Read the model definition and answer for the solid it produces. Units are mm, in the model's axes. A direction names the side the tool comes from. Coordinates: 2 decimals unless noted, no trailing zeros. Loops run counter-clockwise (first coordinate to the right, second up) from the corner with the lowest first, then second, coordinate; pieces in that order, holes last. Notation, with made-up numbers: (51.5, 22) - (110.5, 22) arc R18 ccw to (110.5, 48) - close; hole circle Ø5 at (-13.75, -19.5). An arc over 180 degrees is marked (long way). Use one line per item in the form item = value.
Autodesk Inventor part; units mm, degrees
ref_plane "YZ Plane" through (0, 0, 0) normal (1, 0, 0) x (0, 1, 0)
ref_plane "XZ Plane" through (0, 0, 0) normal (0, 1, 0) x (-1, 0, 0)
ref_plane "XY Plane" through (0, 0, 0) normal (0, 0, 1) x (1, 0, 0)
sketch "Эскиз1" plane through (0, 0, 0) normal (0, 0, 1) x (1, 0, 0)
  line L0 (0, 0) -> (0, 50)
  line L1 (0, 42) -> (4, 42)
  line L2 (4, 42) -> (4, 33)
  line L3 (4, 33) -> (3.5, 33)
  line L4 (3.5, 33) -> (3.5, 31.9)
  line L5 (3.5, 31.9) -> (4, 31.9)
  line L6 (4, 31.9) -> (4, 4)
  line L7 (2, 0) -> (0, 0)
  line L8 (4, 4) -> (3.2, 4)
  line L9 (3.2, 4) -> (2, 0)
  dimension "d0" = 50
  dimension "d2" = 8
  dimension "d3" = 0.5
  dimension "d7" = 9
  dimension "d38" = 1.1
  dimension "d39" = 0.8
  dimension "d40" = 4
  dimension "d41" = 42
revolve "Вращение1" add sketch "Эскиз1" angle 360 about axis through (0, 0, 0) along (0, 1, 0)
hole "Отверстие1" at (0, 0, 0) direction (0, 1, 0) diameter 2.459 depth 10 tip angle 118
chamfer "Фаска1" distance 0.1 angle 45 1 edges at (-4, 42, 0)
sketch "Эскиз2" plane through (0, 42, 0) normal (0, 1, 0) x (1, 0, 0)
  circle A0 centre (0, 0) radius 3.9
  line L0 (1.25, 4.0963) -> (-1.25, 4.0963)
  line L1 (-1.25, 4.0963) -> (-1.25, -4.0963)
  line L2 (-1.25, -4.0963) -> (1.25, -4.0963)
  line L3 (1.25, -4.0963) -> (1.25, 4.0963)
  line L4 (1.25, 4.0963) -> (-1.25, -4.0963) construction
  line L5 (-1.25, 4.0963) -> (1.25, -4.0963) construction
  dimension "d23" = 2.5
extrude "Выдавливание1" cut sketch "Эскиз2" against normal blind 8 contours L3 A0 L1 | A0 L1 L0 L3 | L3 L2 L1 A0
hole "Отверстие2" at (-1.25, 39, 0.2003) direction (-1, 0, 0) diameter 3 end through all both
chamfer "Фаска2" distance 0.3 angle 45 4 edges at (3.8791, 39.9309, -0.9759) (3.8791, 38.0692, -0.9759) (3.6206, 38.9989, 1.7003) (-3.6206, 39.0021, 1.7003)
properties part number "kern"
Item 1: The part is cut by section C-C on z = 0.5. Count the separate pieces of the cut face and the enclosed holes in it, plus the area to 3 significant figures.
Results below:
separate_pieces = 3
enclosed_holes = 0
area = 262 mm²
Item 2: The part is cut by section A-A on y = 24. Give the vertices of the cut face in (x, z), plus the area to 3 significant figures.
Results below:
outline = circle Ø8 at (0, 0)
area = 50.3 mm²
Item 3: The part is cut by section B-B on y = 6. Give the vertices of the cut face in (x, z), plus the area to 3 significant figures.
Results below:
outline = circle Ø8 at (0, 0); hole circle Ø2.46 at (0, 0)
area = 45.5 mm²
Item 4: For a pull along Z with two mould halves and no side action, classify faces 1 (the cylindrical face through (2.458, 39.575, -1.185)), 2 (the cylindrical face through (-0.867, 17.755, -3.905)), 3 (the flat face through (1, 0, -1)) as +Z half, -Z half, draft (parallel to the pull), parting line (faces both ways), or undercut.
Results below:
face_1 = undercut
face_2 = parting line
face_3 = draft
Item 5: Which of the six approach directions +Z, -Z, +X, -X, +Y, -Y give full straight-line access (tool end or side, diameter ignored) to faces 4 (the flat face through (-1.25, 37, 0)), 5 (the cylindrical face through (3.233, 32.442, -1.341)), 6 (the cylindrical face through (0.748, 5.07, 0.976))?
Results below:
face_4 = +Z, -Z, +Y
face_5 = none
face_6 = -Y
Item 6: Find the intervals of material crossed by L1, parallel to X at y = 40.5, z = -1.25; L2, parallel to Z at x = 0, y = 7; L3, parallel to Z at x = -1.5, y = 11, in increasing order.
Results below:
L1 = -3.8 to -1.25, 1.25 to 3.8
L2 = -4 to -1.23, 1.23 to 4
L3 = -3.71 to 3.71
Item 7: Each of these flat-tipped pins is pushed along its axis until it touches: P1, Ø1, axis at x = 1.5, y = 30, coming from the +Z side; P2, Ø0.8, axis at x = -0.5, z = -1.5, coming from the +Y side; P3, Ø3, axis at y = 13, z = 2, coming from the +X side. Where does it stop, or does it pass through?
Results below:
P1 = 3.87
P2 = 34
P3 = 3.97
